```python
from build123d import *

# Parameters (mm, degrees)
EXTRUDE_1_DEPTH     = 10
SKETCH_2_R          = 5
CUT_EXTRUDE_1_DEPTH = 4.5
SKETCH_3_R          = 2
EXTRUDE_2_DEPTH     = 4
SKETCH_4_R          = 1
CUT_EXTRUDE_2_DEPTH = 11
SKETCH_5_R          = 1.95
CUT_EXTRUDE_3_DEPTH = 8
SKETCH_6_R          = 4.25
CUT_EXTRUDE_4_DEPTH = 3


with BuildPart() as part:
    # 草图1 → 凸台-拉伸1 (new body)
    with BuildSketch(Plane(origin=(0, 0, 0), x_dir=(1, 0, 0), z_dir=(0, 1, 0))):
        with BuildLine():
            Line((7.763932023, -2), (-7.763932023, -2))
            ThreePointArc((-7.763932023, -2), (-13, 0), (-7.763932023, 2))
            Line((-7.763932023, 2), (7.763932023, 2))
            ThreePointArc((7.763932023, 2), (13, 0), (7.763932023, -2))
        make_face()
    extrude(amount=EXTRUDE_1_DEPTH)

    # 草图2 → 切除-拉伸1 (cut)
    with BuildSketch(Plane(origin=(0, 10, 0), x_dir=(1, 0, 0), z_dir=(0, 1, 0))):
        with Locations((-10, 0)):
            Circle(SKETCH_2_R)
        with Locations((10, 0)):
            Circle(SKETCH_2_R)
    extrude(amount=-CUT_EXTRUDE_1_DEPTH, mode=Mode.SUBTRACT)

    # 草图3 → 凸台-拉伸2 (add)
    with BuildSketch(Plane(origin=(0, 5.5, 0), x_dir=(1, 0, 0), z_dir=(0, 1, 0))):
        with Locations((-10, 0)):
            Circle(SKETCH_3_R)
        with Locations((10, 0)):
            Circle(SKETCH_3_R)
    extrude(amount=EXTRUDE_2_DEPTH)

    # 草图4 → 切除-拉伸2 (cut, through all)
    with BuildSketch(Plane(origin=(0, 10, 0), x_dir=(1, 0, 0), z_dir=(0, 1, 0))):
        Circle(SKETCH_4_R)
    extrude(amount=-CUT_EXTRUDE_2_DEPTH, mode=Mode.SUBTRACT)

    # 草图5 → 切除-拉伸3 (cut)
    with BuildSketch(Plane(origin=(0, 10, 0), x_dir=(1, 0, 0), z_dir=(0, 1, 0))):
        Circle(SKETCH_5_R)
    extrude(amount=-CUT_EXTRUDE_3_DEPTH, mode=Mode.SUBTRACT)

    # 草图6 → 切除-拉伸4 (cut)
    with BuildSketch(Plane(origin=(0, 10, 0), x_dir=(1, 0, 0), z_dir=(0, 1, 0))):
        Circle(SKETCH_6_R)
    extrude(amount=-CUT_EXTRUDE_4_DEPTH, mode=Mode.SUBTRACT)


solid = part.part
```
Design review of the part built by this model. Coordinates are the model's own, in mm. A direction names the side the tool comes from. Round coordinates to 2 decimals unless told otherwise and drop trailing zeros. Write each loop counter-clockwise with the first axis right and the second up, starting at its lowest first coordinate (ties: lowest second). Pieces come first, ordered by that corner, then holes.
Item 1: We need section B-B on x = 0. Write out the cut boundary in (y, z).
Item 2: For faces 1 (the flat face through (2, 4, 2)), 2 (the cylindrical face through (-1.437, 4.535, -1.318)), 3 (the flat face through (-10, 9.5, 0)), list the 3-axis set-ups (+Z, -Z, +X, -X, +Y, -Y) from which the entire face can be reached by the end or side of a thin tool; tool diameter is ignored.
Item 3: We need section D-D on x = 10. Write out the cut boundary in (y, z).
Item 4: The part is to be moulded in two halves that separate along X. For faces 4 (the cylindrical face through (-13, 3, 0)), 5 (the flat face through (10, 9.5, 0)), say which applies: +X half, -X half, draft (parallel to the pull), parting line (faces both ways), or undercut.
Item 5: Clearance check with flat-ended pins moving along their axes: pin 1 Ø4 at (x, y) = (-2, 2) entering from -Z; pin 2 Ø6 at (x, y) = (-5, 1.5) entering from -Z; pin 3 Ø1 at (x, y) = (7, 2) entering from +Z; pin 4 Ø1.2 at (x, z) = (0, 0) entering from +Y. State where each tip first meets the part, or that it passes through.
Item 6: We need section A-A on z = 0. Write out the cut boundary in (x, y), and give its area (3 significant figures).
Item 7: We need section C-C on y = 7.5. Write out the cut boundary in (x, z).
Item 8: For probe 1 along X at (y, z) = (5.85, 0); probe 2 along X at (y, z) = (0.5, 0); probe 3 along X at (y, z) = (3.45, 0), list the stretches that pass through material, from the lowest coordinate up.
Returned:
1. outline: (0, -2) - (7, -2) - (7, -1.95) - (2, -1.95) - (2, -1) - (0, -1) - close; (0, 1) - (2, 1) - (2, 1.95) - (7, 1.95) - (7, 2) - (0, 2) - close
2. face 1: +Z, +Y, -Y
2. face 2: +Y
2. face 3: +Z, -Z, -X, +Y
3. outline: (0, -3) - (5.5, -3) - (5.5, -2) - (9.5, -2) - (9.5, 2) - (5.5, 2) - (5.5, 3) - (0, 3) - close
4. face 4: undercut
4. face 5: draft
5. pin 1: stops at z = -2
5. pin 2: stops at z = -2.24
5. pin 3: stops at z = 2
5. pin 4: passes through
6. outline: (-13, 0) - (-1, 0) - (-1, 2) - (-1.95, 2) - (-1.95, 7) - (-4.25, 7) - (-4.25, 10) - (-5, 10) - (-5, 5.5) - (-8, 5.5) - (-8, 9.5) - (-12, 9.5) - (-12, 5.5) - (-13, 5.5) - close; (1, 0) - (13, 0) - (13, 5.5) - (12, 5.5) - (12, 9.5) - (8, 9.5) - (8, 5.5) - (5, 5.5) - (5, 10) - (4.25, 10) - (4.25, 7) - (1.95, 7) - (1.95, 2) - (1, 2) - close
6. area: 171 mm2
7. outline: circle Ø4 at (-10, 0); (-5.42, -2) - (-3.75, -2) arc R4.25 cw to (-3.75, 2) - (-5.42, 2) arc R5 cw to start; (3.75, -2) - (5.42, -2) arc R5 cw to (5.42, 2) - (3.75, 2) arc R4.25 cw to start; circle Ø4 at (10, 0)
8. probe 1: x = -12 to -8, -5 to -1.95, 1.95 to 5, 8 to 12
8. probe 2: x = -13 to -1, 1 to 13
8. probe 3: x = -13 to -1.95, 1.95 to 13
